Source: CAD feature listing. Evaluate the final solid. Frame: model axes, mm. A direction names the side the tool comes from. Give positions to 0.01 mm unless a question says otherwise; leave off trailing zeros. Loops run counter-clockwise (first coordinate to the right, second up) from the corner with the lowest first, then second, coordinate; pieces in that order, holes last. Notation, with made-up numbers: (39, 70) -> (45, 70) arc R11 cw to (45, 83) -> close; hole circle Ø3 at (43, 52.5). An arc over 180 degrees is marked (long way). Put each result on its own line as item: value.
```python
from build123d import *
from build123d.topology import SkipClean

# Parameters (mm, degrees)
SKETCH1_W            = 50
SKETCH1_H            = 300
BOSS_EXTRUDE1_DEPTH  = 50
SKETCH2_W            = 50
SKETCH2_H            = 75
CUT_EXTRUDE3_DEPTH   = 50
BOSS_EXTRUDE2_DEPTH  = 50
BOSS_EXTRUDE3_DEPTH  = 100
BOSS_EXTRUDE4_START  = 60
BOSS_EXTRUDE4_DEPTH  = 60
BOSS_EXTRUDE12_DEPTH = 30
SKETCH13_W           = 50
SKETCH13_H           = 150
BOSS_EXTRUDE13_DEPTH = 30
SKETCH14_W           = 30
SKETCH14_H           = 50
BOSS_EXTRUDE14_DEPTH = 120
CUT_EXTRUDE4_DEPTH   = 290
SKETCH17_W           = 50
SKETCH17_H           = 44.956964621
CUT_EXTRUDE5_DEPTH   = 50
SKETCH18_W           = 50
SKETCH18_H           = 50
BOSS_EXTRUDE15_DEPTH = 40
SKETCH19_R           = 15
CUT_EXTRUDE6_DEPTH   = 90


with BuildPart() as part:
    # Sketch1 → Boss-Extrude1 (new body)
    with BuildSketch(Plane.XY):
        with Locations((25, 150)):
            Rectangle(SKETCH1_W, SKETCH1_H)
    extrude(amount=BOSS_EXTRUDE1_DEPTH)

    # Sketch2 → Cut-Extrude3 (cut)
    with BuildSketch(Plane.ZY):
        with Locations((25, 37.5)):
            Rectangle(SKETCH2_W, SKETCH2_H)
    extrude(amount=-CUT_EXTRUDE3_DEPTH, mode=Mode.SUBTRACT)

    # Sketch4 → Boss-Extrude2 (add)
    with BuildSketch(Plane.ZY):
        Polygon((350, 0), (50, 300), (0, 344.956964621), (0, 300), (300, 0), align=None)
    extrude(amount=-BOSS_EXTRUDE2_DEPTH)

    # Sketch5 → Boss-Extrude3 (add)
    with BuildSketch(Plane.XZ):
        with BuildLine():
            ThreePointArc((50, 325), (42.67766953, 342.67766953), (25, 350))
            Line((25, 350), (25, 300))
            ThreePointArc((25, 300), (42.67766953, 307.32233047), (50, 325))
        make_face()
        with BuildLine():
            Line((25, 300), (25, 350))
            ThreePointArc((25, 350), (0, 325), (25, 300))
        make_face()
    extrude(amount=-BOSS_EXTRUDE3_DEPTH)

    # Sketch6 → Boss-Extrude4 (add)
    with BuildSketch(Plane.XZ.offset(BOSS_EXTRUDE4_START)):
        with BuildLine():
            ThreePointArc((50, 325), (42.67766953, 342.67766953), (25, 350))
            Line((25, 350), (25, 300))
            ThreePointArc((25, 300), (42.67766953, 307.32233047), (50, 325))
        make_face()
        with BuildLine():
            Line((25, 300), (25, 350))
            ThreePointArc((25, 350), (0, 325), (25, 300))
        make_face()
    extrude(amount=-BOSS_EXTRUDE4_DEPTH)

    # Sketch9 → Boss-Extrude12 (add)
    with BuildSketch(Plane.XZ.offset(60)):
        Polygon((50, 300), (0, 300), (-150, 300), (-150, 350), (0, 350), (50, 350), (200, 350), (200, 300), align=None)
    extrude(amount=-BOSS_EXTRUDE12_DEPTH)

    # Sketch13 → Boss-Extrude13 (add)
    with SkipClean():  # the faces are left unmerged after this step: merging them gives an invalid solid
        with BuildSketch(Plane.ZY.offset(150)):
            with Locations((325, -105)):
                Rectangle(SKETCH13_W, SKETCH13_H)
        extrude(amount=-BOSS_EXTRUDE13_DEPTH)

    # Sketch14 → Boss-Extrude14 (add)
    with SkipClean():  # the faces are left unmerged after this step: merging them gives an invalid solid
        with BuildSketch(Plane.XZ.offset(60)):
            with Locations((65, 325)):
                Rectangle(SKETCH14_W, SKETCH14_H)
        extrude(amount=BOSS_EXTRUDE14_DEPTH)

    # Sketch15 → Cut-Extrude4 (cut)
    with SkipClean():  # the faces are left unmerged after this step: merging them gives an invalid solid
        with BuildSketch(Plane.ZY.offset(150)):
            with BuildLine():
                ThreePointArc((325, -140), (310, -155), (325, -170))
                Line((325, -170), (325, -140))
            make_face()
            with BuildLine():
                Line((325, -140), (325, -170))
                ThreePointArc((325, -170), (335.606601718, -165.606601718), (340, -155))
                ThreePointArc((340, -155), (335.606601718, -144.393398282), (325, -140))
            make_face()
        extrude(amount=-CUT_EXTRUDE4_DEPTH, mode=Mode.SUBTRACT)

    # Sketch17 → Cut-Extrude5 (cut)
    with SkipClean():  # the faces are left unmerged after this step: merging them gives an invalid solid
        with BuildSketch(Plane.XY):
            with Locations((25, 322.47848231)):
                Rectangle(SKETCH17_W, SKETCH17_H)
        extrude(amount=CUT_EXTRUDE5_DEPTH, mode=Mode.SUBTRACT)

    # Sketch18 → Boss-Extrude15 (add)
    with SkipClean():  # the faces are left unmerged after this step: merging them gives an invalid solid
        with BuildSketch(Plane(origin=(0, 300, 0), x_dir=(1, 0, 0), z_dir=(0, 1, 0))):
            with Locations((25, -25)):
                Rectangle(SKETCH18_W, SKETCH18_H)
        extrude(amount=BOSS_EXTRUDE15_DEPTH)

    # Sketch19 → Cut-Extrude6 (cut)
    with SkipClean():  # the faces are left unmerged after this step: merging them gives an invalid solid
        with BuildSketch(Plane(origin=(50, 0, 0), x_dir=(0, 0, -1), z_dir=(1, 0, 0))):
            with Locations((-25, 320.076220665)):
                Circle(SKETCH19_R)
        extrude(amount=-CUT_EXTRUDE6_DEPTH, mode=Mode.SUBTRACT)


solid = part.part
```
(1) Reachability of faces 4 (the flat face through (5, 0, 344)), 5 (the flat face through (6, 5, 345)), 6 (the flat face through (25, 100, 325)), 7 (the flat face through (44, 0, 305)), 8 (the flat face through (45, 0, 345)) from +Z, -Z, +X, -X, +Y, -Y: full face, straight path, thin tool, end or side. Return the list, or none.
Calculated:
face 4: +Z, -X
face 5: +Z, -X, +Y
face 6: +Z, +X, -X, +Y
face 7: -Z, +X
face 8: +Z, +X
(2) Section B-B on z = 25. Return loops of the section in (x, y).
Calculated:
outline: (0, 75) -> (50, 75) -> (50, 305.08) -> (0, 305.08) -> close; (0, 335.08) -> (50, 335.08) -> (50, 340) -> (0, 340) -> close
(3) First-contact query: P1, Ø25, axis at x = -29, z = 328.5, coming from the -Y side; P2, Ø15, axis at y = -119, z = 333, coming from the +X side; P3, Ø12, axis at x = 18, y = 329.5, coming from the +Z side. Flat tips, straight axial feed; report the tip coordinate or a pass-through.
Calculated:
P1: stops at y = -60
P2: stops at x = 80
P3: stops at z = 50
(4) Section A-A on y = 170. Return loops of the section in (x, z).
Calculated:
outline: (0, 0) -> (50, 0) -> (50, 50) -> (0, 50) -> close; (0, 130) -> (50, 130) -> (50, 180) -> (0, 180) -> close
(5) Draft query along Y for faces 1 (the flat face through (141, -60, 325)), 2 (the flat face through (-150, -106, 325)), 3 (the cylindrical face through (25.35, 334.95, 26.95)). Return one class per face: released by +Y, released by -Y, zero draft, split by the parting line, or undercut.
Calculated:
face 1: released by -Y
face 2: zero draft
face 3: undercut
(6) Line query: probe 1 along Y at (x, z) = (24, 25); probe 2 along Z at (x, y) = (-19.5, -58); probe 3 along X at (y, z) = (238, 101.5). Output: solid intervals per line, ascending. Write a range as from..to.
Calculated:
probe 1: y = 75..305.08, 335.08..340
probe 2: z = 300..350
probe 3: x = 0..50
(7) Section D-D on y = 39. Return loops of the section in (x, z).
Calculated:
outline: (0, 261) -> (50, 261) -> (50, 311) -> (45.71, 311) arc R25 ccw (long way) to (4.29, 311) -> (0, 311) -> close
(8) Section C-C on x = 38.5. Return loops of the section in (y, z).
Calculated:
outline: (-60, 300) -> (-30, 300) -> (-30, 303.96) -> (0, 303.96) -> (0, 300) -> (250, 50) -> (75, 50) -> (75, 0) -> (340, 0) -> (340, 50) -> (300, 50) -> (46.04, 303.96) -> (100, 303.96) -> (100, 346.04) -> (3.96, 346.04) -> (0, 350) -> (0, 346.04) -> (-30, 346.04) -> (-30, 350) -> (-60, 350) -> close; hole circle Ø30 at (320.08, 25)
